The drawing under review shows one solid part. Ordinate dimensions are in mm from its lowest x, y, z. A direction names the side the tool comes from. Give positions to 0.01 mm unless a question says otherwise; leave off trailing zeros. Loops run counter-clockwise (first coordinate to the right, second up) from the corner with the lowest first, then second, coordinate; pieces in that order, holes last. Notation, with made-up numbers: (64, 58) - (109, 58) arc R17 ccw to (109, 74) - close; hole circle Ø9 at (14.25, 0.25). An arc over 180 degrees is marked (long way). One line per item, written item: value. Start each with the question number.
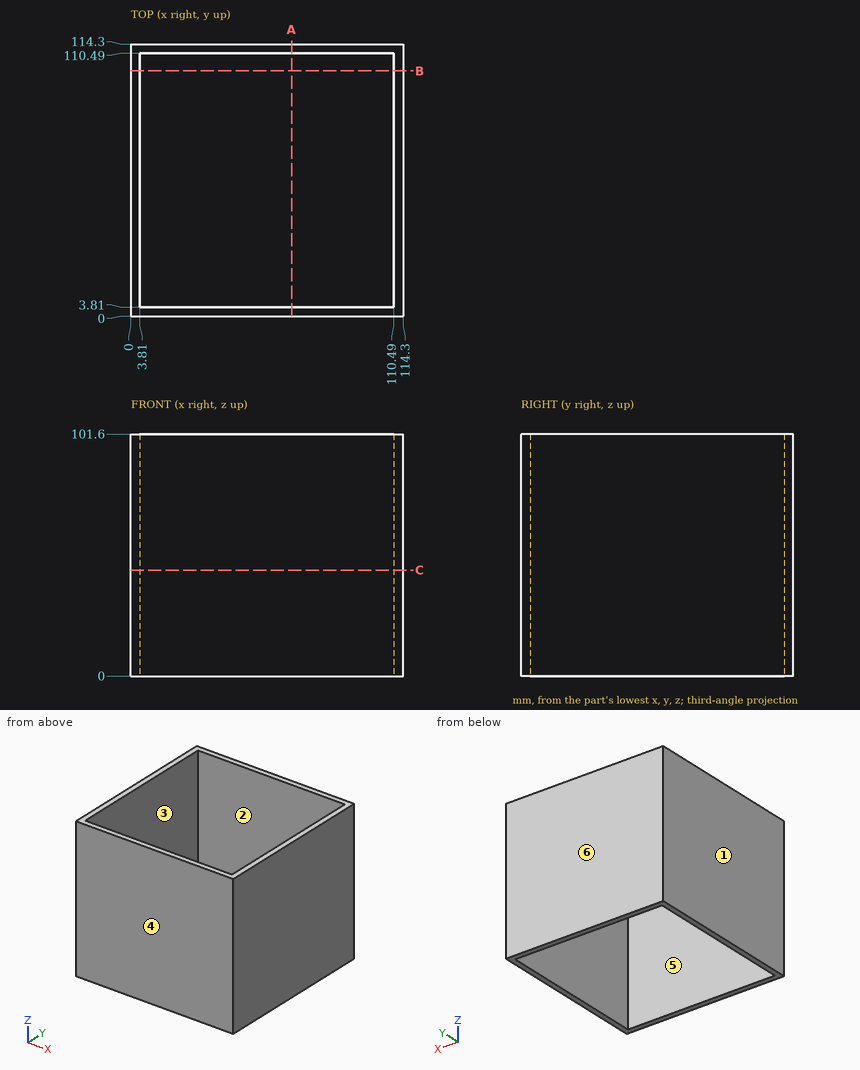
(1) Take a section at A-A on x = 67.5. State the section outline as (y, z) points, and give its area (3 significant figures).
(2) For pin 1 Ø1 at (y, z) = (41, 34) entering from -X, flat-tipped, find the tip position at first contact; note if it passes through.
(3) Machinability: for the marked faces 1 and 2, which of the approach directions +Z, -Z, +X, -X, +Y, -Y give a long, thin tool a straight path to every point of the face, cutting with its end or side? Answer none if there is none.
(4) Draft analysis for pull direction Y (two halves, no side actions). For the marked faces 3, 4, 5 and 6, state which applies: pulls with the +Y half, pulls with the -Y half, needs draft (parallel to the pull), parting line crosses it, or undercut.
(5) Take a section at C-C on z = 44.5. State the section outline as (x, y) points.
(6) To check wall thickness, follow L1, parallel to Y at x = 84, z = 47.5. State the ranges of the line that lie inside material, in increasing order. Write a range as from..to.
Here are the results:
1. outline: (0, 0) - (3.81, 0) - (3.81, 101.6) - (0, 101.6) - close; (110.49, 0) - (114.3, 0) - (114.3, 101.6) - (110.49, 101.6) - close
1. area: 774 mm²
2. pin 1: x = 0
3. face 1: +Z, -Z, -X, +Y, -Y
3. face 2: +Z, -Z
4. face 3: undercut
4. face 4: pulls with the -Y half
4. face 5: undercut
4. face 6: pulls with the +Y half
5. outline: (0, 0) - (114.3, 0) - (114.3, 114.3) - (0, 114.3) - close; hole (3.81, 3.81) - (110.49, 3.81) - (110.49, 110.49) - (3.81, 110.49) - close
6. L1: 0..3.81, 110.49..114.3
